Read the model definition and answer for the solid it produces. Units are mm, in the model's axes. A direction names the side the tool comes from. Coordinates: 2 decimals unless noted, no trailing zeros. Loops run counter-clockwise (first coordinate to the right, second up) from the corner with the lowest first, then second, coordinate; pieces in that order, holes last. Notation, with made-up numbers: (57.25, 53.25) - (65.25, 53.25) arc R20 cw to (65.25, 92.25) - close; hole circle Ø11 at (22, 24.25). An arc over 180 degrees is marked (long way). One line per question, with ' | ' between items. Start each with the question number.
```python
from build123d import *

# Parameters (mm, degrees)
F0_W     = 127
F0_H     = 76.2
F1_DEPTH = 25.4
F3_R     = 12.7
F4_T     = -2.54
F6_D     = 5.1054
F7_ANGLE = 90


with BuildPart() as f1:
    # F0 (on Top) → F1 (new body)
    with BuildSketch(Plane.XY):
        Rectangle(F0_W, F0_H)
    extrude(amount=F1_DEPTH)

    # F3
    f3_edges = [f1.edges().sort_by_distance(p)[0] for p in [
        (-63.5, -38.1, 12.7),
        (-63.5, 38.1, 12.7),
    ]]
    fillet(f3_edges, radius=F3_R)

    # F4
    f4_openings = [f1.faces().sort_by_distance(p)[0] for p in [
        (63.5, 0, 12.7),
    ]]
    offset(amount=F4_T, openings=f4_openings)

    # F6 (through all)
    with Locations(Plane.XY.offset(25.4)):
        with Locations((6.35, 0)):
            Hole(F6_D / 2)


with BuildPart() as f1_1:
    # F7: moved
    add(f1.part.rotate(Axis((63.5, 0, 25.4), (0, 1, 0)), F7_ANGLE))


solid = f1_1.part
```
1) Find the intervals of material crossed by line 1 along X through (y, z) = (20.5, 51); line 2 along Y through (x, z) = (56.5, 74); line 3 along Y through (x, z) = (39.6, 82.55), in increasing order. Write a range as from..to.
2) The part is cut by section A-A on y = 0. Write down the section's boundary in (x, z), and give its area (3 significant figures).
3) Which of the six approach directions +Z, -Z, +X, -X, +Y, -Y give full straight-line access (tool end or side, diameter ignored) to faces 5 (the cylindrical face through (62.21, 2.53, 82.22)), 6 (the flat face through (51, -35.56, 83))?
4) The mould has two halves that part along X. Classify faces 1 (the flat face through (40.64, 0, 89)), 2 (the cylindrical face through (50.942, 32.505, 146.963)), 3 (the flat face through (38.1, 1, 90)), 4 (the flat face through (40, 0, 25.4)): released by +X, released by -X, zero draft, split by the parting line, or undercut.
5) Given pin 1 Ø4 at (y, z) = (0, 82.55) entering from +X; pin 2 Ø1.5 at (x, y) = (56, 29.5) entering from -Z; pin 3 Ø10 at (x, y) = (51.5, 11.5) entering from -Z; pin 4 Ø4 at (x, y) = (60, 28) entering from -Z, each flat-ended and moving along its own axis, determine where each tip first touches the part or whether it passes through.
6) The part is cut by section B-B on z = 82.55. Write down the section's boundary in (x, y).
7) The part is cut by section C-C on z = 119. Write down the section's boundary in (x, y).
8) The part is cut by section D-D on x = 47.25. Write down the section's boundary in (y, z), and give its area (3 significant figures).
Answer below:
1) line 1: 38.1..40.64, 60.96..63.5 | line 2: -38.1..-35.56, 35.56..38.1 | line 3: -38.1..-2.55, 2.55..38.1
2) outline: (38.1, 25.4) - (40.64, 25.4) - (40.64, 80) - (38.1, 80) - close; (38.1, 85.1) - (40.64, 85.1) - (40.64, 149.86) - (60.96, 149.86) - (60.96, 85.1) - (63.5, 85.1) - (63.5, 152.4) - (38.1, 152.4) - close; (60.96, 25.4) - (63.5, 25.4) - (63.5, 80) - (60.96, 80) - close | area: 671 mm2
3) face 5: +X, -X | face 6: -Z
4) face 1: undercut | face 2: undercut | face 3: released by -X | face 4: zero draft
5) pin 1: through | pin 2: z = 148.63 | pin 3: z = 149.86 | pin 4: z = 25.4
6) outline: (38.1, -38.1) - (63.5, -38.1) - (63.5, -2.55) - (60.96, -2.55) - (60.96, -35.56) - (40.64, -35.56) - (40.64, -2.55) - (38.1, -2.55) - close; (38.1, 2.55) - (40.64, 2.55) - (40.64, 35.56) - (60.96, 35.56) - (60.96, 2.55) - (63.5, 2.55) - (63.5, 38.1) - (38.1, 38.1) - close
7) outline: (38.1, -38.1) - (63.5, -38.1) - (63.5, 38.1) - (38.1, 38.1) - close; hole (40.64, -35.56) - (60.96, -35.56) - (60.96, 35.56) - (40.64, 35.56) - close
8) outline: (-38.1, 25.4) - (-35.56, 25.4) - (-35.56, 139.7) arc R10.16 cw to (-25.4, 149.86) - (25.4, 149.86) arc R10.16 cw to (35.56, 139.7) - (35.56, 25.4) - (38.1, 25.4) - (38.1, 139.7) arc R12.7 ccw to (25.4, 152.4) - (-25.4, 152.4) arc R12.7 ccw to (-38.1, 139.7) - close | area: 801 mm2
